```python
from build123d import *

# Parameters (mm, degrees)
SKETCH2_W           = 20
SKETCH2_H           = 20
BOSS_EXTRUDE1_DEPTH = 1
SKETCH3_R           = 5
SKETCH3_R_2         = 1.5
CUT_EXTRUDE1_DEPTH  = 15.177446879
FILLET1_R           = 2
SKETCH4_W           = 15
SKETCH4_H           = 1
BOSS_EXTRUDE2_DEPTH = 5


with BuildPart() as part:
    # Sketch2 → Boss-Extrude1 (new body)
    with BuildSketch(Plane(origin=(0, 0, 0), x_dir=(1, 0, 0), z_dir=(0, 1, 0))):
        Rectangle(SKETCH2_W, SKETCH2_H)
    extrude(amount=BOSS_EXTRUDE1_DEPTH)

    # Sketch3 → Cut-Extrude1 (cut, through all)
    with BuildSketch(Plane(origin=(0, 1, 0), x_dir=(1, 0, 0), z_dir=(0, 1, 0))):
        with Locations(Location((0, 0, 0), (0, 0, 270))):
            Circle(SKETCH3_R)
        with Locations(Location((-8, 8, 0), (0, 0, 270))):
            Circle(SKETCH3_R_2)
        with Locations(Location((8, 8, 0), (0, 0, 270))):
            Circle(SKETCH3_R_2)
    extrude(amount=-CUT_EXTRUDE1_DEPTH, mode=Mode.SUBTRACT)

    # Fillet1
    fillet1_edges = [part.edges().sort_by_distance(p)[0] for p in [
        (10, 0.5, 10),
        (-10, 0.5, 10),
        (-10, 0.5, -10),
        (10, 0.5, -10),
    ]]
    fillet(fillet1_edges, radius=FILLET1_R)

    # Sketch4 → Boss-Extrude2 (add)
    with BuildSketch(Plane.XZ):
        with Locations((0, 9)):
            Rectangle(SKETCH4_W, SKETCH4_H)
    extrude(amount=BOSS_EXTRUDE2_DEPTH)


solid = part.part
```
Source: CAD feature listing. Evaluate the final solid. Frame: model axes, mm. A direction names the side the tool comes from. Give positions to 0.01 mm unless a question says otherwise; leave off trailing zeros. Loops run counter-clockwise (first coordinate to the right, second up) from the corner with the lowest first, then second, coordinate; pieces in that order, holes last. Notation, with made-up numbers: M 27,57 L 69,57 A21 cw 69,67 Z; hole C -27.5,42 d5. An arc over 180 degrees is marked long. Put each result on its own line as item: value.
Q1. Section D-D (x = 2). Return the cut outline in (y, z), and give its area (3 significant figures).
Response values:
outline: M -5,8.5 L 0,8.5 L 0,4.58 L 1,4.58 L 1,10 L 0,10 L 0,9.5 L -5,9.5 Z; M 0,-10 L 1,-10 L 1,-4.58 L 0,-4.58 Z
area: 15.8 mm²
Q2. Reachability of faces 4 (the flat face through (7.5, -2, 9)), 5 (the flat face through (0, -2, 9.5)), 6 (the flat face through (-7.5, -2, 9)), 7 (the flat face through (0, -2, 8.5)) from +Z, -Z, +X, -X, +Y, -Y: full face, straight path, thin tool, end or side. Return the list, or none.
Response values:
face 4: +Z, -Z, +X, -Y
face 5: +Z, +X, -X, -Y
face 6: +Z, -Z, -X, -Y
face 7: -Z, +X, -X, -Y
Q3. Mould query, pull axis Z, two halves, no side actions, for faces 1 (the cylindrical face through (-9.43, 0.51, -9.4)), 2 (the flat face through (-0.1, 0.5, 10)), 3 (the cylindrical face through (-9.464, 0.507, -8.325)). Classes: released by +Z, released by -Z, zero draft, split by the parting line, or undercut.
Response values:
face 1: released by -Z
face 2: released by +Z
face 3: undercut
Q4. Pin query (flat end, axial travel): P1, Ø1.5, axis at x = 6, z = 1, coming from the -Y side; P2, Ø2.5, axis at x = -8, z = -8, coming from the -Y side; P3, Ø0.5, axis at y = -3.5, z = 9, coming from the -X side; P4, Ø1.5, axis at x = -2, y = -3, coming from the -Z side. Return the tip coordinate at first contact, or that it passes through.
Response values:
P1: stops at y = 0
P2: passes through
P3: stops at x = -7.5
P4: stops at z = 8.5
Q5. Line query: probe 1 along X at (y, z) = (0.25, -8); probe 2 along X at (y, z) = (0.5, 0); probe 3 along Z at (x, y) = (3.25, -0.4). Output: solid intervals per line, ascending. Write a range as [from, to].
Response values:
probe 1: x = [-10, -9.5], [-6.5, 6.5], [9.5, 10]
probe 2: x = [-10, -5], [5, 10]
probe 3: z = [8.5, 9.5]
Q6. Section C-C (y = -4.25). Return the cut outline in (x, z).
Response values:
outline: M -7.5,8.5 L 7.5,8.5 L 7.5,9.5 L -7.5,9.5 Z
Q7. Section B-B (x = 0). Return the cut outline in (y, z), and give its area (3 significant figures).
Response values:
outline: M -5,8.5 L 0,8.5 L 0,5 L 1,5 L 1,10 L 0,10 L 0,9.5 L -5,9.5 Z; M 0,-10 L 1,-10 L 1,-5 L 0,-5 Z
area: 15.0 mm²
Q8. Section A-A (z = 0). Return the cut outline in (x, y).
Response values:
outline: M -10,0 L -5,0 L -5,1 L -10,1 Z; M 5,0 L 10,0 L 10,1 L 5,1 Z
